Source: CAD feature listing. Evaluate the final solid. Frame: model axes, mm. Face numbers are marked on the shaded views. A direction names the side the tool comes from. Round coordinates to 2 decimals unless told otherwise and drop trailing zeros. Order: outer loops, then holes, each group sorted by start corner. A loop starts at its lowest first (then second) coordinate and runs counter-clockwise, first axis right, second up. Notation, with made-up numbers: (7.5, 30.25) - (12.5, 30.25) arc R28 cw to (12.5, 63.25) - close; hole circle Ø8 at (49.25, 49.25). An arc over 180 degrees is marked (long way). Use one line per item in the form item = value. Start each with the question number.
Q1. Cut plane B-B, the plane y = 3. Return the cut outline in (x, z), and give its area (3 significant figures).
Q2. Cut plane A-A, the plane x = 0. Return the cut outline in (y, z), and give its area (3 significant figures).
Q3. Cut plane C-C, the plane z = 26.5. Return the cut outline in (x, y), and give its area (3 significant figures).
Q4. Pin query (flat end, axial travel): pin 1 Ø1.8 at (x, y) = (9.64, -11.49) entering from +Z; pin 2 Ø4 at (y, z) = (13.5, 14) entering from -X; pin 3 Ø2 at (x, z) = (3, 14) entering from -Y. Return the tip coordinate at first contact, or that it passes through.
Q5. Ray query, line 1 (X direction, y = 14, z = 32.5); line 2 (Z direction, x = -11.5, y = 11); line 3 (Y direction, x = 0, z = 32). Return the intervals inside material, ascending. Write a range as [from, to].
Q6. Cut plane D-D, the plane y = -7.5. Return the cut outline in (x, z), and give its area (3 significant figures).
Q7. Set-up query: the marked faces 1, 2 and 3. Return all of +Z, -Z, +X, -X, +Y, -Y with unobstructed straight access to the full face (end or side cutting, diameter ignored); none if empty.
from build123d import *

# Parameters (mm, degrees)
SKETCH1_R           = 19
BOSS_EXTRUDE1_DEPTH = 34
SKETCH2_R           = 1.5
CUT_EXTRUDE1_DEPTH  = 6
SKETCH3_R           = 10
BOSS_EXTRUDE2_DEPTH = 5
BOSS_EXTRUDE3_DEPTH = 12


with BuildPart() as part:
    # Sketch1 → Boss-Extrude1 (new body)
    with BuildSketch(Plane.XY):
        Circle(SKETCH1_R)
    extrude(amount=BOSS_EXTRUDE1_DEPTH)

    # Sketch2 → Cut-Extrude1 (cut)
    with BuildSketch(Plane.XY.offset(34)):
        with Locations((-12.990381057, -7.5)):
            Circle(SKETCH2_R)
        with Locations((-14.772116295, -2.604722665)):
            Circle(SKETCH2_R)
        with Locations((0, 15)):
            Circle(SKETCH2_R)
        with Locations((5.13030215, 14.095389312)):
            Circle(SKETCH2_R)
        with Locations((12.990381057, -7.5)):
            Circle(SKETCH2_R)
        with Locations((9.641814145, -11.490666647)):
            Circle(SKETCH2_R)
    extrude(amount=-CUT_EXTRUDE1_DEPTH, mode=Mode.SUBTRACT)

    # Sketch3 → Boss-Extrude2 (add)
    with BuildSketch(Plane.XY.offset(34)):
        Circle(SKETCH3_R)
    extrude(amount=BOSS_EXTRUDE2_DEPTH)

    # Sketch4 → Boss-Extrude3 (add)
    with BuildSketch(Plane.XY.offset(39)):
        with BuildLine():
            ThreePointArc((3, 0), (2.802517077, 1.070466269), (2.236067977, 2))
            Line((2.236067977, 2), (-2.236067977, 2))
            ThreePointArc((-2.236067977, 2), (-1.070466269, -2.802517077), (3, 0))
        make_face()
    extrude(amount=BOSS_EXTRUDE3_DEPTH)


solid = part.part
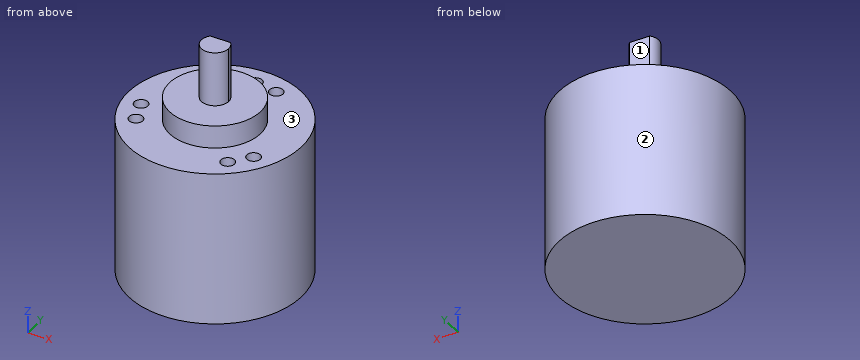
Completed:
q1.outline = (-18.76, 0) - (18.76, 0) - (18.76, 34) - (9.54, 34) - (9.54, 39) - (-9.54, 39) - (-9.54, 34) - (-18.76, 34) - close
q1.area = 1,370 mm2
q2.outline = (-19, 0) - (19, 0) - (19, 34) - (16.5, 34) - (16.5, 28) - (13.5, 28) - (13.5, 34) - (10, 34) - (10, 39) - (2, 39) - (2, 51) - (-3, 51) - (-3, 39) - (-10, 39) - (-10, 34) - (-19, 34) - close
q2.area = 1,430 mm2
q3.outline = circle Ø38 at (0, 0)
q3.area = 1,130 mm2
q4.pin_1 = 28
q4.pin_2 = -15.12
q4.pin_3 = -18.89
q5.line_1 = [-12.85, -1.12], [1.12, 3.63], [6.63, 12.85]
q5.line_2 = [0, 34]
q5.line_3 = [-19, 13.5], [16.5, 19]
q6.outline = (-17.46, 0) - (17.46, 0) - (17.46, 34) - (14.49, 34) - (14.49, 28) - (11.49, 28) - (11.49, 34) - (6.61, 34) - (6.61, 39) - (-6.61, 39) - (-6.61, 34) - (-11.49, 34) - (-11.49, 28) - (-14.49, 28) - (-14.49, 34) - (-17.46, 34) - close
q6.area = 1,220 mm2
q7.face_1 = +Z, +X, -X, +Y
q7.face_2 = +Z, -Z
q7.face_3 = +Z
